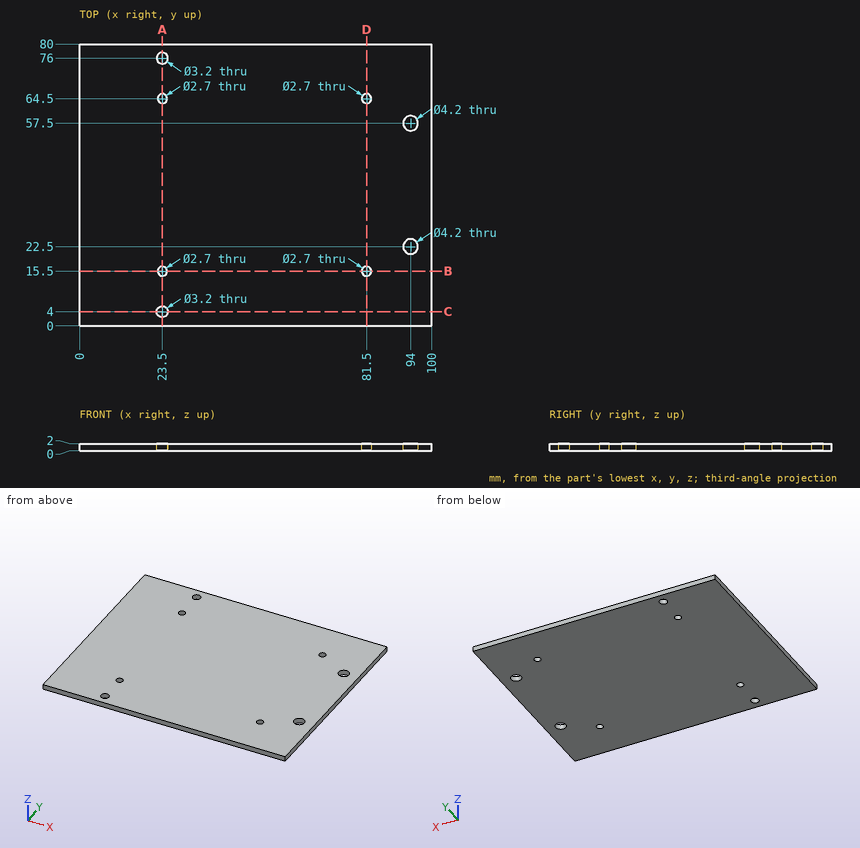
Input: dimensioned drawing with shaded views. Units: mm. Origin: part minimum x, y, z. Give positions to 0.01 mm unless a question says otherwise; leave off trailing zeros. Write each loop counter-clockwise with the first axis right and the second up, starting at its lowest first coordinate (ties: lowest second). Pieces come first, ordered by that corner, then holes. Notation, with made-up numbers: (-39.75, 24.25) -> (-19.75, 24.25) arc R26 ccw to (-19.75, 39.25) -> close; hole circle Ø8 at (40.25, 42.5). An arc over 180 degrees is marked (long way). Answer as a JSON object with one key per item and string values.
1. Contact query for a flat-ended pin moving along its axis: pin 1 (3 mm diameter, centred on x = 23.5, y = 4, fed in from +Z). Output: stop coordinate, or through.
Ans:
{"pin 1": "passes through"}
2. Ray query, probe 1 along Y at (x, z) = (81.5, 0.8); probe 2 along Y at (x, z) = (93.5, 0.35); probe 3 along Y at (x, z) = (23, 0.15). Return the intervals inside material, ascending. Write a range as from..to.
Ans:
{"probe 1": "y = 0..14.15, 16.85..63.15, 65.85..80", "probe 2": "y = 0..20.46, 24.54..55.46, 59.54..80", "probe 3": "y = 0..2.48, 5.52..14.25, 16.75..63.25, 65.75..74.48, 77.52..80"}
3. Cut plane D-D on x = 81.5. Output: boundary loops of the cut face in (y, z), and give its area (3 significant figures).
Ans:
{"outline": "(0, 0) -> (14.15, 0) -> (14.15, 2) -> (0, 2) -> close; (16.85, 0) -> (63.15, 0) -> (63.15, 2) -> (16.85, 2) -> close; (65.85, 0) -> (80, 0) -> (80, 2) -> (65.85, 2) -> close", "area": "149 mm^2"}
4. Cut plane B-B on y = 15.5. Output: boundary loops of the cut face in (x, z).
Ans:
{"outline": "(0, 0) -> (22.15, 0) -> (22.15, 2) -> (0, 2) -> close; (24.85, 0) -> (80.15, 0) -> (80.15, 2) -> (24.85, 2) -> close; (82.85, 0) -> (100, 0) -> (100, 2) -> (82.85, 2) -> close"}
5. Cut plane C-C on y = 4. Output: boundary loops of the cut face in (x, z).
Ans:
{"outline": "(0, 0) -> (21.9, 0) -> (21.9, 2) -> (0, 2) -> close; (25.1, 0) -> (100, 0) -> (100, 2) -> (25.1, 2) -> close"}
6. Cut plane A-A on x = 23.5. Output: boundary loops of the cut face in (y, z), and give its area (3 significant figures).
Ans:
{"outline": "(0, 0) -> (2.4, 0) -> (2.4, 2) -> (0, 2) -> close; (5.6, 0) -> (14.15, 0) -> (14.15, 2) -> (5.6, 2) -> close; (16.85, 0) -> (63.15, 0) -> (63.15, 2) -> (16.85, 2) -> close; (65.85, 0) -> (74.4, 0) -> (74.4, 2) -> (65.85, 2) -> close; (77.6, 0) -> (80, 0) -> (80, 2) -> (77.6, 2) -> close", "area": "136 mm^2"}
